from build123d import *

# Parameters (mm, degrees)
F1_DEPTH = 25
F2_R     = 2
F3_R     = 2


with BuildPart() as f1:
    # F0 (on Front) → F1 (new body)
    with BuildSketch(Plane.XZ):
        Polygon((-12.5, 7.5), (-12.5, 0), (12.5, 0), (12.5, 7.5), (1.25, 20.904757), (1.25, 8.404757), (-1.25, 8.404757), (-1.25, 20.904757), align=None)
    extrude(amount=F1_DEPTH)

    # F2
    f2_edges = [f1.edges().sort_by_distance(p)[0] for p in [
        (12.5, -12.5, 7.5),
        (1.25, -12.5, 20.904757),
        (6.875, 0, 14.202378),
        (6.875, -25, 14.202378),
        (12.5, -12.5, 0),
        (12.5, 0, 3.75),
        (12.5, -25, 3.75),
    ]]
    fillet(f2_edges, radius=F2_R)

    # F3
    f3_edges = [f1.edges().sort_by_distance(p)[0] for p in [
        (-12.5, -12.5, 7.5),
        (-12.5, -12.5, 0),
        (-12.5, 0, 3.75),
        (-12.5, -25, 3.75),
        (-1.25, -12.5, 20.904757),
        (-6.875, 0, 14.202378),
        (-6.875, -25, 14.202378),
    ]]
    fillet(f3_edges, radius=F3_R)


solid = f1.part
CAD build for the part. Positions are in the model's coordinates, mm. A direction names the side the tool comes from. Round coordinates to 2 decimals unless told otherwise and drop trailing zeros. Order: outer loops, then holes, each group sorted by start corner. A loop starts at its lowest first (then second) coordinate and runs counter-clockwise, first axis right, second up. Notation, with made-up numbers: (-1.5, -10) -> (6.5, -10) arc R19 cw to (6.5, 26) -> close; hole circle Ø5 at (-39, 55.25). An arc over 180 degrees is marked (long way). Write each question's results on one line, items separated by ' | '.
1. 3-axis set-ups, long thin cutter, end or side, ignore diameter. For faces 1 (the face through (-1.25, -12, 12)), 2 (the face through (11.93, -24.4, 3.43)): which of +Z, -Z, +X, -X, +Y, -Y reach the whole face in a straight line?
Findings below:
face 1: +Z, +Y, -Y | face 2: +Z, -Z, +X, -Y
2. Pull direction X, two halves, no side cores. Call faces 3 (the face through (0, -12, 8.405)), 4 (the face through (-12.4, -12.6, 7.4)), 5 (the face through (0, -12, 0)): pulls with the +X half, pulls with the -X half, needs draft (parallel to the pull), parting line crosses it, or undercut.
Findings below:
face 3: undercut | face 4: pulls with the -X half | face 5: needs draft
3. Cut at B-B (y = -23.5). Give the cut face in (x, z).
Findings below:
outline: (-12.44, 1.5) arc R2 ccw to (-10.5, 0) -> (10.5, 0) arc R2 ccw to (12.44, 1.5) -> (12.44, 6.77) arc R1.94 ccw to (11.98, 8.02) -> (4.41, 17.04) arc R2 ccw to (1.25, 15.41) -> (1.25, 8.4) -> (-1.25, 8.4) -> (-1.25, 15.41) arc R2 ccw to (-4.41, 17.04) -> (-11.98, 8.02) arc R1.94 ccw to (-12.44, 6.77) -> close
4. Flat gauge pins, fed straight in: P1, Ø4, axis at x = -9.5, y = -7.5, coming from the +Z side; P2, Ø2, axis at y = -18.5, z = 13, coming from the +X side; P3, Ø5.5, axis at y = -17.5, z = 10.5, coming from the -X side. Where does each tip first touch, or does it go through?
Findings below:
P1: stops at z = 13.46 | P2: stops at x = 8.72 | P3: stops at x = -12.24
5. Wall check: line 1 along X through (y, z) = (-15, 10.5); line 2 along X through (y, z) = (-1.75, 13.75); line 3 along Z through (x, y) = (-10.25, -18). Give the ranges that are in metal, low to high. Write a range as [from, to].
Findings below:
line 1: x = [-9.98, -1.25], [1.25, 9.98] | line 2: x = [-7.23, -1.25], [1.25, 7.23] | line 3: z = [0, 10.18]
6. Cut at A-A (y = -5). Give the cut face in (x, z), plus the area to 3 significant figures.
Findings below:
outline: (-12.5, 2) arc R2 ccw to (-10.5, 0) -> (10.5, 0) arc R2 ccw to (12.5, 2) -> (12.5, 6.77) arc R2 ccw to (12.03, 8.06) -> (4.78, 16.7) arc R2 ccw to (1.25, 15.41) -> (1.25, 8.4) -> (-1.25, 8.4) -> (-1.25, 15.41) arc R2 ccw to (-4.78, 16.7) -> (-12.03, 8.06) arc R2 ccw to (-12.5, 6.77) -> close | area: 327 mm²
